from build123d import *

# Parameters (mm, degrees)
PAD015_DEPTH = 20
PAD016_DEPTH = 30
PAD017_DEPTH = 20
PAD018_DEPTH = 30
PAD019_DEPTH = 30
PAD020_DEPTH = 20


with BuildPart() as part:
    # Sketch024 → Pad015 (new body)
    with BuildSketch(Plane.XY):
        with BuildLine():
            ThreePointArc((0, 38.4), (-27.1529, 27.1529), (-38.4, 0))
            Line((-38.4, 0), (-32.1, 0))
            ThreePointArc((-27.838774, 15.981636), (-31.016404, 8.269987), (-32.1, 0))
            ThreePointArc((-20.653618, 24.573116), (-28.541936, 23.869954), (-27.838774, 15.981636))
            ThreePointArc((-5.6, 31.607752), (-13.589873, 29.081358), (-20.653618, 24.573116))
            ThreePointArc((0, 37.207752), (-3.959798, 35.56755), (-5.6, 31.607752))
            Line((0, 38.4), (0, 37.207752))
        make_face()
    pad015 = extrude(amount=-PAD015_DEPTH)

    # Sketch025 → Pad016 (join)
    with BuildSketch(Plane.XY):
        with BuildLine():
            ThreePointArc((-1.8e-05, 36.6), (-25.880117, 25.880104), (-36.6, 0))
            Line((-36.6, 0), (-38.4, 0))
            ThreePointArc((0, 38.4), (-27.152903, 27.152903), (-38.4, 0))
            Line((0, 38.4), (-1.8e-05, 36.6))
        make_face()
    pad016 = extrude(amount=PAD016_DEPTH)

    # Sketch026 → Pad017 (join)
    with BuildSketch(Plane.XY):
        with BuildLine():
            ThreePointArc((-32.1, 0), (-23.735101, -21.611455), (-3, -31.959506))
            Line((-3, -31.959506), (-3.588785, -38.231932))
            ThreePointArc((-38.4, 0), (-28.393391, -25.852956), (-3.588785, -38.231932))
            Line((-38.4, 0), (-32.1, 0))
        make_face()
    pad017 = extrude(amount=-PAD017_DEPTH)

    # Sketch027 → Pad018 (join)
    with BuildSketch(Plane.XY):
        with BuildLine():
            ThreePointArc((0, 38.4), (-38.35796, 1.796359), (-3.588785, -38.231932))
            Line((-3.420561, -36.43981), (-3.588785, -38.231932))
            ThreePointArc((-1.8e-05, 36.6), (-36.559931, 1.712146), (-3.420561, -36.43981))
            Line((0, 38.4), (-1.8e-05, 36.6))
        make_face()
    pad018 = extrude(amount=PAD018_DEPTH)

    # Mirrored003: Pad018, Pad017, Pad016, Pad015 across Sketch027 V_Axis
    add(pad018.mirror(Plane(origin=(0, 0, 0), x_dir=(0, 0, 1), z_dir=(1, 0, 0))))
    add(pad017.mirror(Plane(origin=(0, 0, 0), x_dir=(0, 0, 1), z_dir=(1, 0, 0))))
    add(pad016.mirror(Plane(origin=(0, 0, 0), x_dir=(0, 0, 1), z_dir=(1, 0, 0))))
    add(pad015.mirror(Plane(origin=(0, 0, 0), x_dir=(0, 0, 1), z_dir=(1, 0, 0))))

    # Sketch028 → Pad019 (join)
    with BuildSketch(Plane.XY):
        with BuildLine():
            ThreePointArc((-6.188785, -37.898007), (-4.891635, -38.087162), (-3.588785, -38.231932))
            Line((-3.588785, -38.231932), (-3.588785, -43.231932))
            Line((-3.588785, -43.231932), (-8.588785, -43.231932))
            Line((-8.588785, -43.231932), (-8.588785, -42.071032))
            Line((-8.588785, -42.071032), (-7.588785, -41.231932))
            Line((-7.588785, -41.231932), (-5.588785, -41.231932))
            Line((-5.588785, -41.231932), (-5.588785, -38.498007))
            Line((-5.588785, -38.498007), (-6.188785, -37.898007))
        make_face()
    pad019 = extrude(amount=PAD019_DEPTH)

    # Sketch028 → Pad020 (join)
    with BuildSketch(Plane.XY):
        with BuildLine():
            ThreePointArc((-6.188785, -37.898007), (-4.891635, -38.087162), (-3.588785, -38.231932))
            Line((-3.588785, -38.231932), (-3.588785, -43.231932))
            Line((-3.588785, -43.231932), (-8.588785, -43.231932))
            Line((-8.588785, -43.231932), (-8.588785, -42.071032))
            Line((-8.588785, -42.071032), (-7.588785, -41.231932))
            Line((-7.588785, -41.231932), (-5.588785, -41.231932))
            Line((-5.588785, -41.231932), (-5.588785, -38.498007))
            Line((-5.588785, -38.498007), (-6.188785, -37.898007))
        make_face()
    pad020 = extrude(amount=-PAD020_DEPTH)

    # Mirrored004: Pad019, Pad020 across Sketch028 V_Axis
    add(pad019.mirror(Plane(origin=(0, 0, 0), x_dir=(0, 0, 1), z_dir=(1, 0, 0))))
    add(pad020.mirror(Plane(origin=(0, 0, 0), x_dir=(0, 0, 1), z_dir=(1, 0, 0))))


with BuildPart() as part_1:
    # Body020 placement: moved
    add(part.part.moved(Location((127, 0, 0))))


solid = part_1.part
Part model, mm, in its own coordinate system. A direction names the side the tool comes from. Give positions to 0.01 mm unless a question says otherwise; leave off trailing zeros. Write each loop counter-clockwise with the first axis right and the second up, starting at its lowest first coordinate (ties: lowest second). Pieces come first, ordered by that corner, then holes.
1) Cut at B-B on y = -20. Write the cut outline in (x, z).
Resolved:
outline: (94.22, -20) - (101.89, -20) - (101.89, 0) - (96.35, 0) - (96.35, 30) - (94.22, 30) - close; (152.11, -20) - (159.78, -20) - (159.78, 30) - (157.65, 30) - (157.65, 0) - (152.11, 0) - close
2) Pin check, flat tips, straight feed: pin 1 (2 mm diameter, centred on x = 146, z = 24.5, fed in from +Y); pin 2 (5 mm diameter, centred on x = 154.5, z = 0.5, fed in from -Y); pin 3 (1 mm diameter, centred on x = 120.5, z = 10, fed in from +Y). Stop position of each tip, or through.
Resolved:
pin 1: stops at y = 33.92
pin 2: stops at y = -29.15
pin 3: stops at y = 37.93
3) Which spindle directions (+Z, -Z, +X, -X, +Y, -Y) get a long thin tool onto all of the face, cutting with end or side? Do faces 1 (the face through (113.517, 29.131, -9.86)), 2 (the face through (99, 24, 0)), 3 (the face through (120, -41.232, 5)), 4 (the face through (97, -13, 0)), 5 (the face through (134, -41.232, 5)). Say none if no direction does.
Resolved:
face 1: +Z, -Z
face 2: -Z
face 3: +Z, -Z, -X
face 4: +Z
face 5: +Z, -Z, +X
4) Cut at A-A on z = 17. Write the cut outline in (x, y), then the cut area to 3 significant figures.
Resolved:
outline: (88.6, 0) arc R38.4 ccw to (120.81, -37.9) - (121.41, -38.5) - (121.41, -41.23) - (119.41, -41.23) - (118.41, -42.07) - (118.41, -43.23) - (123.41, -43.23) - (123.41, -38.23) - (123.58, -36.44) arc R36.6 cw (long way) to (130.42, -36.44) - (130.59, -38.23) - (130.59, -43.23) - (135.59, -43.23) - (135.59, -42.07) - (134.59, -41.23) - (132.59, -41.23) - (132.59, -38.5) - (133.19, -37.9) arc R38.4 ccw to (127, 38.4) arc R38.4 ccw to start
area: 443 mm2
5) Two-plate mould, pull along X, no slides. Class faces 6 (the face through (130.29, -35.05, -9.86)), 7 (the face through (121.411, -40, 5)), 8 (the face through (112.6, -29.4, -20)), 9 (the face through (163.515, 2.492, 14.79)): released by +X, released by -X, zero draft, split by the parting line, or undercut.
Resolved:
face 6: undercut
face 7: released by -X
face 8: zero draft
face 9: undercut
6) Cut at C-C on x = 105. Write the cut outline in (y, z).
Resolved:
outline: (-31.47, -20) - (-23.38, -20) - (-23.38, 0) - (-29.25, 0) - (-29.25, 30) - (-31.47, 30) - close; (25.41, -20) - (31.47, -20) - (31.47, 30) - (29.25, 30) - (29.25, 0) - (25.41, 0) - close
7) Probe L1, parallel to X at y = -1, z = 7; L2, parallel to Y at x = 133, z = -5; L3, parallel to X at y = -39, z = 16.5. List the from-to ranges inside material, lowest first.
Resolved:
L1: x = 88.61 to 90.41, 163.59 to 165.39
L2: y = -43.23 to -41.23, -38.09 to -31.53, 31.53 to 37.93
L3: x = 121.41 to 123.41, 130.59 to 132.59
